from build123d import *
from build123d.topology import SkipClean

# Parameters (mm, degrees)
ESQUISSE1_R                  = 4.45
BOSS_EXTRU_1_DEPTH           = 1.5
ESQUISSE1_2_R                = 5.95
ESQUISSE1_2_R_2              = 4.45
EXTRU_MINCE1_DEPTH           = 35
ESQUISSE2_R                  = 5.95
ESQUISSE2_R_2                = 4.45
BOSS_EXTRU_2_DEPTH           = 3
ESQUISSE4_W                  = 28
ESQUISSE4_H                  = 38
ESQUISSE4_R                  = 3.05
BOSS_EXTRU_3_DEPTH           = 2
CONG_1_R                     = 10
ESQUISSE5_R                  = 4.45
ENL_V_MAT_EXTRU_1_DEPTH      = 10
ENL_V_MAT_EXTRU_4_DEPTH      = 49.455159684
ENL_V_MAT_EXTRU_4_DEPTH_BACK = 49.455159684
ESQUISSE8_W                  = 5
ESQUISSE8_H                  = 3


with BuildPart() as part:
    # Esquisse1 → Boss.-Extru.1 (new body)
    with BuildSketch(Plane.XY):
        Circle(ESQUISSE1_R)
    extrude(amount=BOSS_EXTRU_1_DEPTH)

    # Esquisse1<2> → Extru.-Mince1 (add)
    with BuildSketch(Plane.XY):
        Circle(ESQUISSE1_2_R)
        Circle(ESQUISSE1_2_R_2, mode=Mode.SUBTRACT)
    extrude(amount=EXTRU_MINCE1_DEPTH)

    # Esquisse2 → Boss.-Extru.2 (add)
    # profile 1 of 3: a face of its own
    with BuildSketch(Plane.XY.offset(35)):
        with BuildLine():
            Line((9.677371186, 3.358041833), (1.677371186, 5.708671115))
            ThreePointArc((1.677371186, 5.708671115), (4.76355217, 3.565258858), (5.95, 0))
            ThreePointArc((5.95, 0), (4.76355217, -3.565258858), (1.677371186, -5.708671115))
            Line((1.677371186, -5.708671115), (9.677371186, -3.358041833))
            ThreePointArc((9.677371186, -3.358041833), (11.492771765, -2.097211093), (12.190682253, 0))
            ThreePointArc((12.190682253, 0), (11.492771765, 2.097211093), (9.677371186, 3.358041833))
        make_face()
    # profile 2 of 3: a face of its own
    with BuildSketch(Plane.XY.offset(35)):
        with BuildLine():
            ThreePointArc((-1.677371186, -5.708671115), (-5.95, 0), (-1.677371186, 5.708671115))
            Line((-1.677371186, 5.708671115), (-9.677371186, 3.358041833))
            ThreePointArc((-9.677371186, 3.358041833), (-11.492771765, 2.097211093), (-12.190682253, 0))
            ThreePointArc((-12.190682253, 0), (-11.492771765, -2.097211093), (-9.677371186, -3.358041833))
            Line((-9.677371186, -3.358041833), (-1.677371186, -5.708671115))
        make_face()
    # profile 3 of 3: a face of its own
    with BuildSketch(Plane.XY.offset(35)):
        with Locations(Location((0, 0, 0), (0, 0, 106.374299713))):
            Circle(ESQUISSE2_R)
        Circle(ESQUISSE2_R_2, mode=Mode.SUBTRACT)
    extrude(amount=BOSS_EXTRU_2_DEPTH)

    # Esquisse4 → Boss.-Extru.3 (add)
    # profile 1 of 4: a face of its own
    with BuildSketch(Plane(origin=(0, -5, 0), x_dir=(1, 0, 0), z_dir=(0, 1, 0))):
        with Locations((14, -19)):
            Rectangle(ESQUISSE4_W, ESQUISSE4_H)
        with Locations(Location((21.5, -10, 0), (0, 0, 270))):
            Circle(ESQUISSE4_R, mode=Mode.SUBTRACT)
    # profile 2 of 4: a face of its own
    with BuildSketch(Plane(origin=(0, -5, 0), x_dir=(1, 0, 0), z_dir=(0, 1, 0))):
        with Locations((-14, -19)):
            Rectangle(ESQUISSE4_W, ESQUISSE4_H)
        with Locations(Location((-21.5, -10, 0), (0, 0, 270))):
            Circle(ESQUISSE4_R, mode=Mode.SUBTRACT)
    # profile 3 of 4: a face of its own
    with BuildSketch(Plane(origin=(0, -5, 0), x_dir=(1, 0, 0), z_dir=(0, 1, 0))):
        with Locations((-14, -19)):
            Rectangle(ESQUISSE4_W, ESQUISSE4_H)
        with Locations(Location((-21.5, -10, 0), (0, 0, 270))):
            Circle(ESQUISSE4_R, mode=Mode.SUBTRACT)
    # profile 4 of 4: a face of its own
    with BuildSketch(Plane(origin=(0, -5, 0), x_dir=(1, 0, 0), z_dir=(0, 1, 0))):
        with Locations((14, -19)):
            Rectangle(ESQUISSE4_W, ESQUISSE4_H)
        with Locations(Location((21.5, -10, 0), (0, 0, 270))):
            Circle(ESQUISSE4_R, mode=Mode.SUBTRACT)
    extrude(amount=-BOSS_EXTRU_3_DEPTH)

    # Congé1
    # the kernel refuses this fillet: 10 mm, written as the material it adds along each edge
    with BuildSketch(Plane(origin=(-3.225290685, -5, 64.801871004), x_dir=(-0.33303824301553137, 0.9429133198174304, 0), z_dir=(0, 0, -1))) as cong_1_piece_1_section:
        with BuildLine():
            CenterArc((13.399198301, -7.90985002), CONG_1_R, 127.722343038, 71.730945551)
            Line((3.970065103, -11.24023245), (0, 0))
            ThreePointArc((0, 0), (3.640421456, -1.243639238), (7.280842913, 0))
        make_face()
    cong_1_piece_1 = extrude(amount=64.801871004, mode=Mode.PRIVATE)
    cong_1_piece_1 = split(cong_1_piece_1, bisect_by=Plane(origin=(-7.500746377, -3.487839575, 38), z_dir=(0, 0, -1)), keep=Keep.TOP, mode=Mode.PRIVATE)
    add(cong_1_piece_1)
    with BuildSketch(Plane(origin=(3.225290685, -5, 64.801871004), x_dir=(0.3330382430155311, 0.9429133198174307, 0), z_dir=(0, 0, -1))) as cong_1_piece_2_section:
        with BuildLine():
            CenterArc((13.399198301, 7.90985002), CONG_1_R, 160.546711411, 71.730945551)
            Line((3.970065103, 11.24023245), (0, 0))
            ThreePointArc((0, 0), (3.640421456, 1.243639238), (7.280842913, 0))
        make_face()
    cong_1_piece_2 = extrude(amount=64.801871004, mode=Mode.PRIVATE)
    cong_1_piece_2 = split(cong_1_piece_2, bisect_by=Plane(origin=(7.500746377, -3.487839575, 38), z_dir=(0, 0, -1)), keep=Keep.TOP, mode=Mode.PRIVATE)
    add(cong_1_piece_2)

    # Esquisse5 → Enlèv. mat.-Extru.1 (cut)
    with SkipClean():  # the faces are left unmerged after this step: merging them gives an invalid solid
        with BuildSketch(Plane(origin=(0, 0, 0), x_dir=(-1, 0, 0), z_dir=(0, 0, -1))):
            Circle(ESQUISSE5_R)
        extrude(amount=-ENL_V_MAT_EXTRU_1_DEPTH, mode=Mode.SUBTRACT)
    add(part.part.scale(1), mode=Mode.REPLACE)  # the faces are merged on a copy

    # Esquisse8 → Enlèv. mat.-Extru.4 (cut, two sides: drawn at the far end of the back side and taken through both)
    with BuildSketch(Plane(origin=(0, -5, 0), x_dir=(1, 0, 0), z_dir=(0, 1, 0)).offset(-ENL_V_MAT_EXTRU_4_DEPTH_BACK)):
        with Locations((-11, -4)):
            Rectangle(ESQUISSE8_W, ESQUISSE8_H)
        with Locations((11, -4)):
            Rectangle(ESQUISSE8_W, ESQUISSE8_H)
    extrude(amount=ENL_V_MAT_EXTRU_4_DEPTH + ENL_V_MAT_EXTRU_4_DEPTH_BACK, mode=Mode.SUBTRACT)


solid = part.part
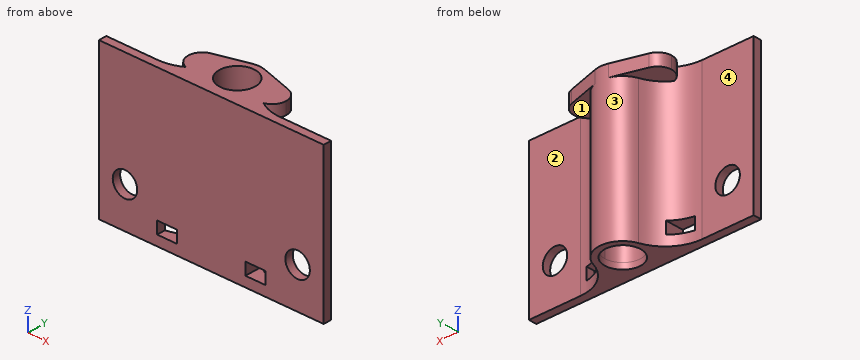
For this review, take the finished solid that the model builds, in its own axes (mm). Face numbers are marked on the shaded views. A direction names the side the tool comes from. Coordinates: 2 decimals unless noted, no trailing zeros. Order: outer loops, then holes, each group sorted by start corner. A loop starts at its lowest first (then second) coordinate and runs counter-clockwise, first axis right, second up. Notation, with made-up numbers: (85, 35.25) - (124, 35.25) arc R25 ccw to (124, 52.25) - close; hole circle Ø8 at (74.25, 1.25). An arc over 180 degrees is marked (long way). Answer as CSV lines item,"result". Start each with the question number.
1) To check wall thickness, follow line 1 along X through (y, z) = (-6.15, 10); line 2 along Y through (x, z) = (0, 27); line 3 along Y through (x, z) = (-18, 24). State the ranges of each line that lie inside material, in increasing order. Write a range as [from, to].
2) Add section B-B (z = 23). State the section outline as (x, y) points.
3) Machinability: for the marked faces 1, 2, 3 and 4, which of the approach directions +Z, -Z, +X, -X, +Y, -Y give a long, thin tool a straight path to every point of the face, cutting with its end or side? Answer none if there is none.
4) Insertion check: P1, Ø3.5, axis at y = -4, z = 3.5, coming from the -X side; P2, Ø1.5, axis at y = 2.5, z = 26, coming from the -X side; P3, Ø4, axis at x = 22, z = 21, coming from the +Y side. Each pin has a flat end and moves straight along its axis. Give the tip position at first contact, or say it passes through.
5) Add section A-A (x = 0). State the section outline as (y, z) points, then the cut area to 3 significant figures.
6) Add section C-C (x = -10.5). State the section outline as (y, z) points.
7) Add section D-D (z = 12). State the section outline as (x, y) points, then the cut area to 3 significant figures.
Result:
1,line 1,"[-28, -24.55], [-18.45, 18.45], [24.55, 28]"
1,line 2,"[-7, -4.45], [4.45, 5.95]"
1,line 3,"[-7, -5]"
2,outline,"(-28, -7) - (28, -7) - (28, -5) - (15.15, -5) arc R10 cw to (5.65, 1.87) arc R5.95 ccw to (-5.65, 1.87) arc R10 cw to (-15.15, -5) - (-28, -5) - close; hole circle Ø8.9 at (0, 0)"
3,face 1,"-Z, +X, +Y"
3,face 2,"+Z, -Z, +X, +Y"
3,face 3,"-Z, +Y"
3,face 4,"+Z, -Z, -X, +Y"
4,P1,"x = -28"
4,P2,"x = -5.69"
4,P3,"y = -5"
5,outline,"(-7, 0) - (-4.45, 0) - (-4.45, 38) - (-7, 38) - close; (4.45, 0) - (5.95, 0) - (5.95, 38) - (4.45, 38) - close"
5,area,"154 mm^2"
6,outline,"(-7, 0) - (-3.86, 0) - (-3.86, 2.5) - (-7, 2.5) - close; (-7, 5.5) - (-3.86, 5.5) - (-3.86, 38) - (-7, 38) - close; (-3, 35) - (3, 35) - (3, 38) - (-3, 38) - close"
7,outline,"(-28, -7) - (-23.8, -7) - (-23.8, -5) - (-28, -5) - close; (-19.2, -7) - (19.2, -7) - (19.2, -5) - (15.15, -5) arc R10 cw to (5.65, 1.87) arc R5.95 ccw to (-5.65, 1.87) arc R10 cw to (-15.15, -5) - (-19.2, -5) - close; (23.8, -7) - (28, -7) - (28, -5) - (23.8, -5) - close; hole circle Ø8.9 at (0, 0)"
7,area,"178 mm^2"
